```python
from build123d import *

# Parameters (mm, degrees)
F1_R     = 1.6
F2_DEPTH = 2


with BuildPart() as f2:
    # F1 (on Front) → F2 (new body)
    with BuildSketch(Plane.XZ):
        with BuildLine():
            Line((47.136039, 58), (10.863961, 58))
            ThreePointArc((10.863961, 58), (9.141886, 57.657458), (7.681981, 56.681981))
            Line((7.681981, 56.681981), (1.318019, 50.318019))
            ThreePointArc((1.318019, 50.318019), (0.342542, 48.858114), (0, 47.136039))
            Line((0, 47.136039), (0, 10.863961))
            ThreePointArc((0, 10.863961), (0.342542, 9.141886), (1.318019, 7.681981))
            Line((1.318019, 7.681981), (7.681981, 1.318019))
            ThreePointArc((7.681981, 1.318019), (9.141886, 0.342542), (10.863961, 0))
            Line((10.863961, 0), (46.928932, 0))
            ThreePointArc((46.928932, 0), (48.842349, 0.380602), (50.464466, 1.464466))
            Line((50.464466, 1.464466), (56.681981, 7.681981))
            ThreePointArc((56.681981, 7.681981), (57.657458, 9.141886), (58, 10.863961))
            Line((58, 10.863961), (58, 47.136039))
            ThreePointArc((58, 47.136039), (57.657458, 48.858114), (56.681981, 50.318019))
            Line((56.681981, 50.318019), (50.318019, 56.681981))
            ThreePointArc((50.318019, 56.681981), (48.858114, 57.657458), (47.136039, 58))
        make_face()
        with Locations((7.786797, 7.786797)):
            Circle(F1_R, mode=Mode.SUBTRACT)
        with BuildLine():
            ThreePointArc((7.197009, 13.56066), (5.562323, 13.235501), (4.636348, 14.62132))
            Line((4.636348, 14.62132), (4.636348, 23))
            ThreePointArc((4.636348, 23), (5.075688, 24.06066), (6.136348, 24.5))
            Line((6.136348, 24.5), (9.136348, 24.5))
            ThreePointArc((9.136348, 24.5), (13.636348, 29), (9.136348, 33.5))
            Line((9.136348, 33.5), (6.136348, 33.5))
            ThreePointArc((6.136348, 33.5), (5.075688, 33.93934), (4.636348, 35))
            Line((4.636348, 35), (4.636348, 43.37868))
            ThreePointArc((4.636348, 43.37868), (5.562323, 44.764499), (7.197009, 44.43934))
            Line((7.197009, 44.43934), (21.575688, 30.06066))
            ThreePointArc((21.575688, 30.06066), (22.015028, 29), (21.575688, 27.93934))
            Line((21.575688, 27.93934), (7.197009, 13.56066))
        make_face(mode=Mode.SUBTRACT)
        with Locations((18.393398, 18.393398)):
            Circle(F1_R, mode=Mode.SUBTRACT)
        with Locations((29, 9.136348)):
            Circle(F1_R, mode=Mode.SUBTRACT)
        with BuildLine():
            Line((33.5, 6.136348), (33.5, 9.136348))
            ThreePointArc((33.5, 9.136348), (29, 13.636348), (24.5, 9.136348))
            Line((24.5, 9.136348), (24.5, 6.136348))
            ThreePointArc((24.5, 6.136348), (24.06066, 5.075688), (23, 4.636348))
            Line((23, 4.636348), (14.62132, 4.636348))
            ThreePointArc((14.62132, 4.636348), (13.235501, 5.562323), (13.56066, 7.197009))
            Line((13.56066, 7.197009), (27.93934, 21.575688))
            ThreePointArc((27.93934, 21.575688), (29, 22.015028), (30.06066, 21.575688))
            Line((30.06066, 21.575688), (44.43934, 7.197009))
            ThreePointArc((44.43934, 7.197009), (44.764499, 5.562323), (43.37868, 4.636348))
            Line((43.37868, 4.636348), (35, 4.636348))
            ThreePointArc((35, 4.636348), (33.93934, 5.075688), (33.5, 6.136348))
        make_face(mode=Mode.SUBTRACT)
        with Locations((50.213203, 7.786797)):
            Circle(F1_R, mode=Mode.SUBTRACT)
        with Locations((39.606602, 18.393398)):
            Circle(F1_R, mode=Mode.SUBTRACT)
        with BuildLine():
            ThreePointArc((50.802991, 44.43934), (52.437677, 44.764499), (53.363652, 43.37868))
            Line((53.363652, 43.37868), (53.363652, 35))
            ThreePointArc((53.363652, 35), (52.924312, 33.93934), (51.863652, 33.5))
            Line((51.863652, 33.5), (48.863652, 33.5))
            ThreePointArc((48.863652, 33.5), (44.363652, 29), (48.863652, 24.5))
            Line((48.863652, 24.5), (51.863652, 24.5))
            ThreePointArc((51.863652, 24.5), (52.924312, 24.06066), (53.363652, 23))
            Line((53.363652, 23), (53.363652, 14.62132))
            ThreePointArc((53.363652, 14.62132), (52.437677, 13.235501), (50.802991, 13.56066))
            Line((50.802991, 13.56066), (36.424312, 27.93934))
            ThreePointArc((36.424312, 27.93934), (35.984972, 29), (36.424312, 30.06066))
            Line((36.424312, 30.06066), (50.802991, 44.43934))
        make_face(mode=Mode.SUBTRACT)
        with Locations((9.136348, 29)):
            Circle(F1_R, mode=Mode.SUBTRACT)
        with Locations((18.393398, 39.606602)):
            Circle(F1_R, mode=Mode.SUBTRACT)
        with Locations((7.786797, 50.213203)):
            Circle(F1_R, mode=Mode.SUBTRACT)
        with Locations((29, 29)):
            Circle(F1_R, mode=Mode.SUBTRACT)
        with Locations((39.606602, 39.606602)):
            Circle(F1_R, mode=Mode.SUBTRACT)
        with Locations((48.863652, 29)):
            Circle(F1_R, mode=Mode.SUBTRACT)
        with BuildLine():
            ThreePointArc((13.56066, 50.802991), (13.235501, 52.437677), (14.62132, 53.363652))
            Line((14.62132, 53.363652), (23, 53.363652))
            ThreePointArc((23, 53.363652), (24.06066, 52.924312), (24.5, 51.863652))
            Line((24.5, 51.863652), (24.5, 48.863652))
            ThreePointArc((24.5, 48.863652), (29, 44.363652), (33.5, 48.863652))
            Line((33.5, 48.863652), (33.5, 51.863652))
            ThreePointArc((33.5, 51.863652), (33.93934, 52.924312), (35, 53.363652))
            Line((35, 53.363652), (43.37868, 53.363652))
            ThreePointArc((43.37868, 53.363652), (44.764499, 52.437677), (44.43934, 50.802991))
            Line((44.43934, 50.802991), (30.06066, 36.424312))
            ThreePointArc((30.06066, 36.424312), (29, 35.984972), (27.93934, 36.424312))
            Line((27.93934, 36.424312), (13.56066, 50.802991))
        make_face(mode=Mode.SUBTRACT)
        with Locations((29, 48.863652)):
            Circle(F1_R, mode=Mode.SUBTRACT)
        with Locations((50.213203, 50.213203)):
            Circle(F1_R, mode=Mode.SUBTRACT)
    extrude(amount=F2_DEPTH)


solid = f2.part
```
Verification items for the finished model (mm, model axes). A direction names the side the tool comes from. Give positions to 0.01 mm unless a question says otherwise; leave off trailing zeros. Loops run counter-clockwise (first coordinate to the right, second up) from the corner with the lowest first, then second, coordinate; pieces in that order, holes last.
1. Section check B-B, the plane x = 29. Enter the section's corners in (y, z), then the cut area to 3 significant figures.
2. Set-up check for faces 4 (the flat face through (54, -1, 53)), 5 (the cylindrical face through (35.985, -0.986, 28.984)): record each of +Z, -Z, +X, -X, +Y, -Y from which the full face is reachable in a straight line by a thin tool's end or side.
3. Mould release check, pull along Z, two halves, no side actions. Record for faces 1 (the flat face through (58, -1, 29)), 2 (the cylindrical face through (44.755, -0.986, 52.46)), 3 (the flat face through (4, -1, 5)): released by +Z, released by -Z, zero draft, split by the parting line, or undercut.
4. Section check D-D, the plane y = -0.5. Count the separate pieces of the cut face and the enclosed holes in it, then the cut area to 3 significant figures.
5. Section check A-A, the plane z = 29. Enter the section's corners in (x, y).
6. Thickness scan on line 1 (Z direction, x = 9, y = -0.3); line 2 (X direction, y = -0.4, z = 32.5); line 3 (X direction, y = -0.9, z = 48.5). Record the ranges inside material, lowest first.
7. Section check C-C, the plane z = 12. Enter the section's corners in (x, y).
8. Go/stop test with flat-tipped pins: pin 1 Ø1 at (x, y) = (7, -1) entering from +Z; pin 2 Ø0.6 at (y, z) = (-1, 51) entering from +X; pin 3 Ø1 at (x, y) = (50, -1) entering from +Z; pin 4 Ø3 at (x, z) = (9.14, 29) entering from -Y. Record where each tip stops, or that it passes through.
Geometry says:
1. outline: (-2, 0) - (0, 0) - (0, 7.54) - (-2, 7.54) - close; (-2, 10.74) - (0, 10.74) - (0, 13.64) - (-2, 13.64) - close; (-2, 22.02) - (0, 22.02) - (0, 27.4) - (-2, 27.4) - close; (-2, 30.6) - (0, 30.6) - (0, 35.98) - (-2, 35.98) - close; (-2, 44.36) - (0, 44.36) - (0, 47.26) - (-2, 47.26) - close; (-2, 50.46) - (0, 50.46) - (0, 58) - (-2, 58) - close
1. area: 63.3 mm2
2. face 4: +Z, +X, +Y, -Y
2. face 5: +Y, -Y
3. face 1: zero draft
3. face 2: undercut
3. face 3: released by -Z
4. separate pieces: 1
4. enclosed holes: 17
4. area: 2,120 mm2
5. outline: (0, -2) - (7.54, -2) - (7.54, 0) - (0, 0) - close; (10.74, -2) - (13.64, -2) - (13.64, 0) - (10.74, 0) - close; (22.02, -2) - (27.4, -2) - (27.4, 0) - (22.02, 0) - close; (30.6, -2) - (35.98, -2) - (35.98, 0) - (30.6, 0) - close; (44.36, -2) - (47.26, -2) - (47.26, 0) - (44.36, 0) - close; (50.46, -2) - (58, -2) - (58, 0) - (50.46, 0) - close
6. line 1: z = 0.4 to 6.74, 8.83 to 15.36, 24.5 to 27.41, 30.59 to 33.5, 42.64 to 49.17, 51.26 to 57.6
6. line 2: x = 0 to 11.96, 19.14 to 38.86, 46.04 to 58
6. line 3: x = 0.21 to 15.86, 24.51 to 27.44, 30.56 to 33.49, 42.14 to 57.79
7. outline: (0, -2) - (18.36, -2) - (18.36, 0) - (0, 0) - close; (25.53, -2) - (32.47, -2) - (32.47, 0) - (25.53, 0) - close; (39.64, -2) - (58, -2) - (58, 0) - (39.64, 0) - close
8. pin 1: stops at z = 56.5
8. pin 2: stops at x = 56.3
8. pin 3: stops at z = 57.33
8. pin 4: passes through
